Geometry check sheet. Reference: the model listing, model coordinates, mm. Give positions to 0.01 mm unless a question says otherwise; leave off trailing zeros. Loops run counter-clockwise (first coordinate to the right, second up) from the corner with the lowest first, then second, coordinate; pieces in that order, holes last.
1. Cross-section at A-A, the plane y = 0. Record the cut outline in (x, z).
2. Material ranges on L1, parallel to X at y = -14, z = 12.5; L2, parallel to X at y = 16.5, z = 10; L3, parallel to Y at x = -11.5, z = 23, recorded low to high.
3. Release check for a two-part mould opening along Y. For faces 1 (the flat face through (30, 10, 63.125)), 2 (the flat face through (0, 0, 2.5)), 3 (the conical face through (-6.008, 27.057, 30.151)) record: +Y half, -Y half, draft (parallel to the pull), parting line (faces both ways), or undercut.
4. Go/stop test with flat-tipped pins: pin 1 Ø4 at (y, z) = (17, 35.5) entering from +X; pin 2 Ø12 at (x, y) = (2.5, 14.5) entering from +Z; pin 3 Ø4 at (x, z) = (18.5, 55) entering from +Y; pin 4 Ø1 at (x, y) = (10, 9.5) entering from -Z. Record where each tip stops, or that it passes through.
5. Cross-section at D-D, the plane z = 41. Record the cut outline in (x, y), plus the area to 3 significant figures.
6. Cross-section at C-C, the plane z = 23. Record the cut outline in (x, y).
from build123d import *

# Parameters (mm, degrees)
F2_T = -2.5
F4_R = 2.5


with BuildPart() as f1:
    # F0 (on Front) → F1 (revolve)
    with BuildSketch(Plane.XZ):
        with BuildLine():
            ThreePointArc((13.84601, 0), (20.476051, 2.420071), (23.98807, 8.542155))
            Line((23.98807, 8.542155), (33.404892, 63.125353))
            Line((33.404892, 63.125353), (0, 63.125353))
            Line((0, 63.125353), (0, 0))
            Line((0, 0), (13.84601, 0))
        make_face()
    revolve(axis=Axis((0, 0, 30.873057), (0, 0, -1)))

    # F2
    f2_openings = [f1.faces().sort_by_distance(p)[0] for p in [
        (0, 0, 63.125353),
    ]]
    offset(amount=F2_T, openings=f2_openings)


with BuildPart() as f5:
    # F5: sweep along a path in F3
    with BuildLine(Plane.XZ) as f5_path:
        Line((25.372773, 17.402936), (44.32266, 35.468507))
        ThreePointArc((44.32266, 35.468507), (45.10088, 49.073565), (31.577616, 50.754206))
    # F4 (on Top) → F5 (sweep)
    with BuildSketch(Plane.XY):
        with Locations((58.820363, 16.743207)):
            Circle(F4_R)
    sweep(path=f5_path.line)


solid = f1.part
Result:
1. outline: (-33.4, 63.13) - (-23.99, 8.54) arc R10.29 ccw to (-13.85, 0) - (13.85, 0) arc R10.29 ccw to (23.99, 8.54) - (33.4, 63.13) - (30.87, 63.13) - (21.52, 8.97) arc R7.79 cw to (13.85, 2.5) - (-13.85, 2.5) arc R7.79 cw to (-21.52, 8.97) - (-30.87, 63.13) - close
2. L1: x = -20.31 to -17.14, 17.14 to 20.31
2. L2: x = -17.76 to -14.1, 14.1 to 17.76
2. L3: y = -23.86 to -21, 21 to 23.86
3. face 1: draft
3. face 2: undercut
3. face 3: parting line
4. pin 1: stops at x = 24.46
4. pin 2: stops at z = 6.61
4. pin 3: stops at y = 27.49
4. pin 4: stops at z = 0
5. outline: circle Ø59.18 at (0, 0); hole circle Ø54.1 at (0, 0)
5. area: 451 mm2
6. outline: circle Ø52.96 at (0, 0); hole circle Ø47.89 at (0, 0)
